Model file for the job. Use its own axes, mm. Round coordinates to 2 decimals unless told otherwise and drop trailing zeros. Order: outer loops, then holes, each group sorted by start corner. A loop starts at its lowest first (then second) coordinate and runs counter-clockwise, first axis right, second up. Notation, with made-up numbers: (59.5, 80.25) - (106.5, 80.25) arc R28 ccw to (106.5, 107.25) - close; hole circle Ø9 at (88, 61.5). An arc over 180 degrees is marked (long way). Use one line per item in the form item = value.
from build123d import *

# Parameters (mm, degrees)
SKETCH1_R           = 2.75
BOSS_EXTRUDE1_DEPTH = 15.5
CHAMFER1_SIZE       = 0.5
BOSS_EXTRUDE2_START = -3
BOSS_EXTRUDE2_DEPTH = 3
CIRPATTERN1_START   = 12
CIRPATTERN1_DEPTH   = 3


# Read off the part's stored shape, not the designer's step: CirPattern1
with BuildPart() as part:
    # Sketch1 → Boss-Extrude1 (new body)
    with BuildSketch(Plane(origin=(0, 0, 0), x_dir=(0, 0, -1), z_dir=(1, 0, 0))):
        Circle(SKETCH1_R)
    extrude(amount=BOSS_EXTRUDE1_DEPTH)

    # Chamfer1
    chamfer1_edges = [part.edges().sort_by_distance(p)[0] for p in [
        (15.5, 0, 2.75),
    ]]
    chamfer(chamfer1_edges, length=CHAMFER1_SIZE)

    # Sketch2 → Boss-Extrude2 (add)
    with BuildSketch(Plane(origin=(15, 0, 0), x_dir=(0, 0, -1), z_dir=(1, 0, 0)).offset(BOSS_EXTRUDE2_START)):
        with BuildLine():
            Line((0, 2.85), (-0.058089283, 2.749386411))
            ThreePointArc((-0.058089283, 2.749386411), (0, 2.75), (0.058089283, 2.749386411))
            Line((0.058089283, 2.749386411), (0, 2.85))
        make_face()
    extrude(amount=BOSS_EXTRUDE2_DEPTH)

    # CirPattern1 outline → CirPattern1 (add)
    with BuildSketch(Plane.YZ.offset(CIRPATTERN1_START)):
        with BuildLine():
            Line((-1.425, -2.351993835), (-1.425, -2.468172401))
            Line((-1.425, -2.468172401), (-1.324386411, -2.410083118))
            ThreePointArc((-1.324386411, -2.410083118), (-1.375, -2.38156986), (-1.425, -2.351993835))
        make_face()
        with BuildLine():
            ThreePointArc((-0.655483627, -2.670737953), (-0.711752374, -2.656296022), (-0.767703504, -2.640668728))
            Line((-0.767703504, -2.640668728), (-0.737634279, -2.752888605))
            Line((-0.737634279, -2.752888605), (-0.655483627, -2.670737953))
        make_face()
        with BuildLine():
            Line((-2.015254326, -2.015254326), (-1.903034449, -1.985185101))
            ThreePointArc((-1.903034449, -1.985185101), (-1.944543648, -1.944543648), (-1.985185101, -1.903034449))
            Line((-1.985185101, -1.903034449), (-2.015254326, -2.015254326))
        make_face()
        with BuildLine():
            ThreePointArc((0.058089283, -2.749386411), (0, -2.75), (-0.058089283, -2.749386411))
            Line((-0.058089283, -2.749386411), (0, -2.85))
            Line((0, -2.85), (0.058089283, -2.749386411))
        make_face()
        with BuildLine():
            Line((-2.468172401, -1.425), (-2.351993835, -1.425))
            ThreePointArc((-2.351993835, -1.425), (-2.38156986, -1.375), (-2.410083118, -1.324386411))
            Line((-2.410083118, -1.324386411), (-2.468172401, -1.425))
        make_face()
        with BuildLine():
            ThreePointArc((0.767703504, -2.640668728), (0.711752374, -2.656296022), (0.655483627, -2.670737953))
            Line((0.655483627, -2.670737953), (0.737634279, -2.752888605))
            Line((0.737634279, -2.752888605), (0.767703504, -2.640668728))
        make_face()
        with BuildLine():
            Line((-2.752888605, -0.737634279), (-2.640668728, -0.767703504))
            ThreePointArc((-2.640668728, -0.767703504), (-2.656296022, -0.711752374), (-2.670737953, -0.655483627))
            Line((-2.670737953, -0.655483627), (-2.752888605, -0.737634279))
        make_face()
        with BuildLine():
            ThreePointArc((1.425, -2.351993835), (1.375, -2.38156986), (1.324386411, -2.410083118))
            Line((1.324386411, -2.410083118), (1.425, -2.468172401))
            Line((1.425, -2.468172401), (1.425, -2.351993835))
        make_face()
        with BuildLine():
            Line((-2.85, 0), (-2.749386411, -0.058089283))
            ThreePointArc((-2.749386411, -0.058089283), (-2.75, 0), (-2.749386411, 0.058089283))
            Line((-2.749386411, 0.058089283), (-2.85, 0))
        make_face()
        with BuildLine():
            ThreePointArc((1.985185101, -1.903034449), (1.944543648, -1.944543648), (1.903034449, -1.985185101))
            Line((1.903034449, -1.985185101), (2.015254326, -2.015254326))
            Line((2.015254326, -2.015254326), (1.985185101, -1.903034449))
        make_face()
        with BuildLine():
            Line((-2.752888605, 0.737634279), (-2.670737953, 0.655483627))
            ThreePointArc((-2.670737953, 0.655483627), (-2.656296022, 0.711752374), (-2.640668728, 0.767703504))
            Line((-2.640668728, 0.767703504), (-2.752888605, 0.737634279))
        make_face()
        with BuildLine():
            ThreePointArc((2.410083118, -1.324386411), (2.38156986, -1.375), (2.351993835, -1.425))
            Line((2.351993835, -1.425), (2.468172401, -1.425))
            Line((2.468172401, -1.425), (2.410083118, -1.324386411))
        make_face()
        with BuildLine():
            Line((-2.468172401, 1.425), (-2.410083118, 1.324386411))
            ThreePointArc((-2.410083118, 1.324386411), (-2.38156986, 1.375), (-2.351993835, 1.425))
            Line((-2.351993835, 1.425), (-2.468172401, 1.425))
        make_face()
        with BuildLine():
            ThreePointArc((2.670737953, -0.655483627), (2.656296022, -0.711752374), (2.640668728, -0.767703504))
            Line((2.640668728, -0.767703504), (2.752888605, -0.737634279))
            Line((2.752888605, -0.737634279), (2.670737953, -0.655483627))
        make_face()
        with BuildLine():
            Line((-2.015254326, 2.015254326), (-1.985185101, 1.903034449))
            ThreePointArc((-1.985185101, 1.903034449), (-1.944543648, 1.944543648), (-1.903034449, 1.985185101))
            Line((-1.903034449, 1.985185101), (-2.015254326, 2.015254326))
        make_face()
        with BuildLine():
            Line((-1.425, 2.468172401), (-1.425, 2.351993835))
            ThreePointArc((-1.425, 2.351993835), (-1.375, 2.38156986), (-1.324386411, 2.410083118))
            Line((-1.324386411, 2.410083118), (-1.425, 2.468172401))
        make_face()
        with BuildLine():
            ThreePointArc((2.640668728, 0.767703504), (2.656296022, 0.711752374), (2.670737953, 0.655483627))
            Line((2.670737953, 0.655483627), (2.752888605, 0.737634279))
            Line((2.752888605, 0.737634279), (2.640668728, 0.767703504))
        make_face()
        with BuildLine():
            Line((-0.737634279, 2.752888605), (-0.767703504, 2.640668728))
            ThreePointArc((-0.767703504, 2.640668728), (-0.711752374, 2.656296022), (-0.655483627, 2.670737953))
            Line((-0.655483627, 2.670737953), (-0.737634279, 2.752888605))
        make_face()
        with BuildLine():
            ThreePointArc((2.351993835, 1.425), (2.38156986, 1.375), (2.410083118, 1.324386411))
            Line((2.410083118, 1.324386411), (2.468172401, 1.425))
            Line((2.468172401, 1.425), (2.351993835, 1.425))
        make_face()
        with BuildLine():
            Line((0, 2.85), (-0.058089283, 2.749386411))
            ThreePointArc((-0.058089283, 2.749386411), (0, 2.75), (0.058089283, 2.749386411))
            Line((0.058089283, 2.749386411), (0, 2.85))
        make_face()
        with BuildLine():
            ThreePointArc((1.903034449, 1.985185101), (1.944543648, 1.944543648), (1.985185101, 1.903034449))
            Line((1.985185101, 1.903034449), (2.015254326, 2.015254326))
            Line((2.015254326, 2.015254326), (1.903034449, 1.985185101))
        make_face()
        with BuildLine():
            Line((0.737634279, 2.752888605), (0.655483627, 2.670737953))
            ThreePointArc((0.655483627, 2.670737953), (0.711752374, 2.656296022), (0.767703504, 2.640668728))
            Line((0.767703504, 2.640668728), (0.737634279, 2.752888605))
        make_face()
        with BuildLine():
            ThreePointArc((1.324386411, 2.410083118), (1.375, 2.38156986), (1.425, 2.351993835))
            Line((1.425, 2.351993835), (1.425, 2.468172401))
            Line((1.425, 2.468172401), (1.324386411, 2.410083118))
        make_face()
    extrude(amount=CIRPATTERN1_DEPTH)


solid = part.part
(1) Slice it at A-A on x = 7.75. Give the cut face in (y, z), then the cut area to 3 significant figures.
Report:
outline = circle Ø5.5 at (0, 0)
area = 23.8 mm2
(2) Probe probe 1 along Y at (x, z) = (12.5, -0.1); probe 2 along Z at (x, y) = (10, -1.9). List the from-to ranges inside material, lowest first. Write a range as [from, to].
Report:
probe_1 = [-2.75, 2.75]
probe_2 = [-1.99, 1.99]
(3) Pin check, flat tips, straight feed: pin 1 (1 mm diameter, centred on x = 5, z = -2, fed in from -Y); pin 2 (3 mm diameter, centred on x = 6.5, z = 1.5, fed in from +Y); pin 3 (2 mm diameter, centred on x = 11, y = -0.5, fed in from -Z). Stop position of each tip, or through.
Report:
pin_1 = -2.3
pin_2 = 2.75
pin_3 = -2.75
